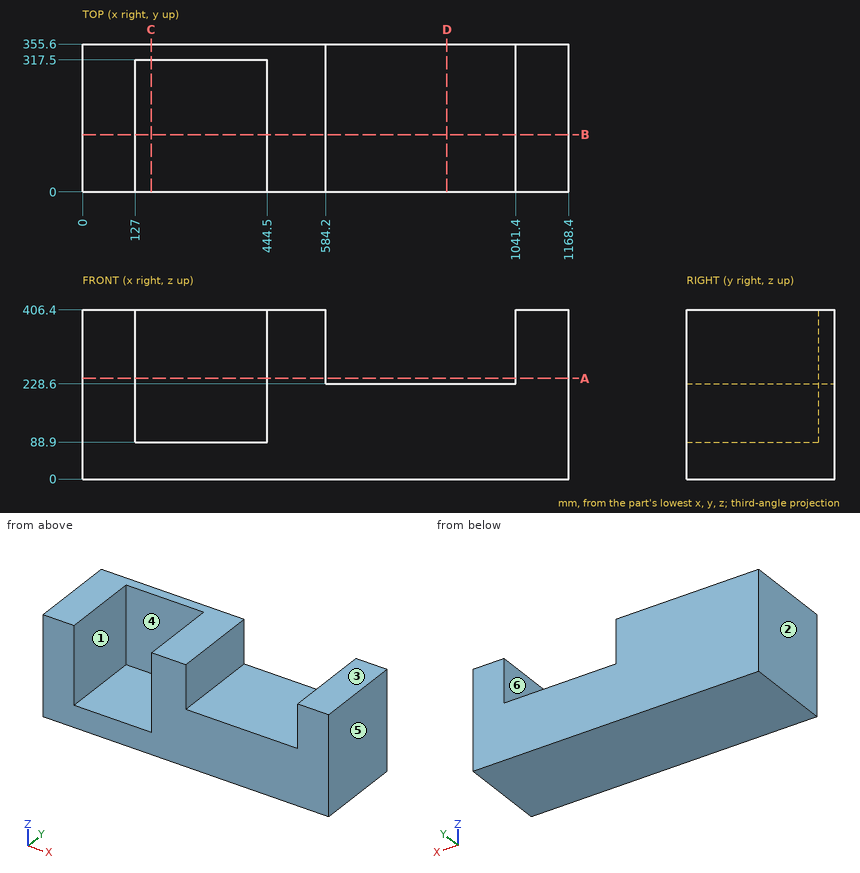
Part print with two shaded views. Sizes in mm from the minimum x, y, z corner. A direction names the side the tool comes from. Coordinates: 2 decimals unless noted, no trailing zeros. Write each loop counter-clockwise with the first axis right and the second up, starting at its lowest first coordinate (ties: lowest second). Pieces come first, ordered by that corner, then holes. Notation, with made-up numbers: (23, 28.25) - (79, 28.25) arc R23 cw to (79, 55.25) - close; hole circle Ø2 at (47, 2.25). An arc over 180 degrees is marked (long way). Put each result on its own line as item: value.
1. 3-axis set-ups, long thin cutter, end or side, ignore diameter. For the marked faces 4, 5 and 6: which of +Z, -Z, +X, -X, +Y, -Y reach the whole face in a straight line?
Final values:
face 4: +Z, -Y
face 5: +Z, -Z, +X, +Y, -Y
face 6: +Z, +Y, -Y
2. Band-saw the part on C-C (x = 165). Write the cut outline in (y, z).
Final values:
outline: (0, 0) - (355.6, 0) - (355.6, 406.4) - (317.5, 406.4) - (317.5, 88.9) - (0, 88.9) - close
3. Probe line 1 along X through (y, z) = (205.5, 366); line 2 along X through (y, z) = (82, 167); line 3 along Z through (x, y) = (400, 260.5). List the from-to ranges inside material, lowest first. Write a range as [from, to].
Final values:
line 1: x = [0, 127], [444.5, 584.2], [1041.4, 1168.4]
line 2: x = [0, 127], [444.5, 1168.4]
line 3: z = [0, 88.9]
4. Band-saw the part on D-D (x = 876). Write the cut outline in (y, z).
Final values:
outline: (0, 0) - (355.6, 0) - (355.6, 228.6) - (0, 228.6) - close
5. Band-saw the part on B-B (y = 138). Write the cut outline in (x, z).
Final values:
outline: (0, 0) - (1168.4, 0) - (1168.4, 406.4) - (1041.4, 406.4) - (1041.4, 228.6) - (584.2, 228.6) - (584.2, 406.4) - (444.5, 406.4) - (444.5, 88.9) - (127, 88.9) - (127, 406.4) - (0, 406.4) - close
6. Two-plate mould, pull along X, no slides. Class the marked faces 1, 2 and 3: +X half, -X half, draft (parallel to the pull), parting line (faces both ways), or undercut.
Final values:
face 1: undercut
face 2: -X half
face 3: draft
7. Flat gauge pins, fed straight in: pin 1 Ø5 at (x, y) = (164, 180) entering from +Z; pin 2 Ø1.5 at (x, z) = (735.5, 192) entering from -Y. Where does each tip first touch, or does it go through?
Final values:
pin 1: stops at z = 88.9
pin 2: stops at y = 0
8. Band-saw the part on A-A (z = 242). Write the cut outline in (x, y).
Final values:
outline: (0, 0) - (127, 0) - (127, 317.5) - (444.5, 317.5) - (444.5, 0) - (584.2, 0) - (584.2, 355.6) - (0, 355.6) - close; (1041.4, 0) - (1168.4, 0) - (1168.4, 355.6) - (1041.4, 355.6) - close
